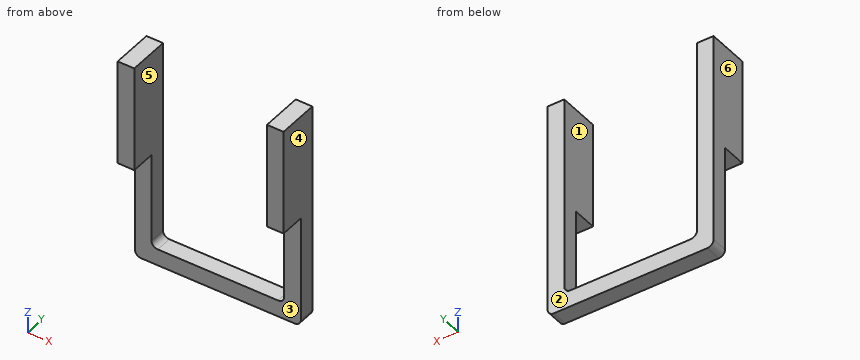
from build123d import *

# Parameters (mm, degrees)
F1_DEPTH = 0.8
F2_R     = 0.3
F3_W     = 0.8
F3_H     = 5.1
F4_DEPTH = 1.2


with BuildPart() as f1:
    # F0 (on Front) → F1 (new body)
    with BuildSketch(Plane.XZ):
        Polygon((3.2, 0), (0, 0), (0, -0.8), (4, -0.8), (4, 9.7), (3.2, 9.7), align=None)
    extrude(amount=F1_DEPTH)

    # F2
    f2_edges = [f1.edges().sort_by_distance(p)[0] for p in [
        (3.2, -0.4, 0),
        (4, -0.4, -0.8),
    ]]
    fillet(f2_edges, radius=F2_R)

    # F3 (on face) → F4 (join)
    with BuildSketch(Plane.XZ.offset(0.8)):
        with Locations((3.6, 7.15)):
            Rectangle(F3_W, F3_H)
    extrude(amount=F4_DEPTH)

    # F5: F1 across face


with BuildPart() as f1_1:
    add(f1.part)
    add(f1.part.mirror(Plane(origin=(0, -0.4, -0.4), x_dir=(0, -1, 0), z_dir=(-1, 0, 0))))


solid = f1_1.part
Check sheet for the modelled part. Datum: model origin and axes. Units: mm. Face numbers are marked on the shaded views. A direction names the side the tool comes from. Coordinates: 2 decimals unless noted, no trailing zeros. Write each loop counter-clockwise with the first axis right and the second up, starting at its lowest first coordinate (ties: lowest second). Pieces come first, ordered by that corner, then holes. Notation, with made-up numbers: M 58.5,58 L 91.5,58 A30 cw 91.5,91 Z; hole C -1.75,16.25 d1. An arc over 180 degrees is marked long. Answer as CSV lines item,"result".
Q1. Material ranges on probe 1 along X at (y, z) = (-0.55, 8); probe 2 along Z at (x, y) = (1, -0.2), recorded low to high. Write a range as from..to.
Check result:
probe 1,"-4..-3.2, 3.2..4"
probe 2,"-0.8..0"
Q2. Cross-section at A-A (z = 0.5). Record the boundary of the cut face in (x, y), then the cut area to 3 significant figures.
Check result:
outline,"M -4,-0.8 L -3.2,-0.8 L -3.2,0 L -4,0 Z; M 3.2,-0.8 L 4,-0.8 L 4,0 L 3.2,0 Z"
area,"1.28 mm^2"
Q3. Mould release check, pull along X, two halves, no side actions. Record for the marked faces 4, 5 and 6: released by +X, released by -X, zero draft, split by the parting line, or undercut.
Check result:
face 4,"released by +X"
face 5,"undercut"
face 6,"released by -X"
Q4. Cross-section at B-B (y = -1.7). Record the boundary of the cut face in (x, z), then the cut area to 3 significant figures.
Check result:
outline,"M -4,4.6 L -3.2,4.6 L -3.2,9.7 L -4,9.7 Z; M 3.2,4.6 L 4,4.6 L 4,9.7 L 3.2,9.7 Z"
area,"8.16 mm^2"
Q5. Set-up check for the marked faces 1, 2 and 3: record each of +Z, -Z, +X, -X, +Y, -Y from which the full face is reachable in a straight line by a thin tool's end or side.
Check result:
face 1,"+Z, +Y, -Y"
face 2,"+Z, -Z, +X, -X, +Y"
face 3,"-Z, +X, -X, -Y"
Q6. Cross-section at C-C (x = 2). Record the boundary of the cut face in (y, z).
Check result:
outline,"M -0.8,-0.8 L 0,-0.8 L 0,0 L -0.8,0 Z"
